Work out the finished part from the listing and answer in its coordinate system (mm). A direction names the side the tool comes from. Round coordinates to 2 decimals unless told otherwise and drop trailing zeros. Loops run counter-clockwise (first coordinate to the right, second up) from the corner with the lowest first, then second, coordinate; pieces in that order, holes last. Notation, with made-up numbers: (-6, -4.5) - (28, -4.5) arc R29 cw to (28, 17.5) - close; hole circle Ø11 at (55.25, 7). An arc over 180 degrees is marked (long way). Answer as CSV lines item,"result". Start each with the question number.
Q1. Each of these flat-tipped pins is pushed along its axis until it touches: pin 1 Ø4 at (x, y) = (35.15, 35.15) entering from +Z; pin 2 Ø1.7 at (x, y) = (14.63, -8.44) entering from -Z. Where does it stop, or does it pass through?
Q2. Section A-A on y = 9 is taken. Write down the section's boundary in (x, z), then the cut area to 3 significant figures.
Q3. Section B-B on x = -10 is taken. Write down the section's boundary in (y, z), then the cut area to 3 significant figures.
Q4. For faces 1 (the face through (-24.041, -17.546, 0.805)), 2 (the face through (-1, 1, 0)), determine the directions among +Z, -Z, +X, -X, +Y, -Y from which every point of the face is accessible in a straight line to the end or side of a thin tool.
Q5. Straight lines are drawn through the part: L1, parallel to Y at x = 0, z = 1; L2, parallel to Y at x = 7, z = 0.1; L3, parallel to X at y = 8.5, z = 1.4. For each, find the intervals that lie inside material, in ascending order. Write a range as [from, to].
Q6. Section D-D on y = -50 is taken. Write down the section's boundary in (x, z).
Q7. Section C-C on z = 1.1 is taken. Count the separate pieces of the cut face and the enclosed holes in it, then the cut area to 3 significant figures.
Q8. The mould has two halves that part along Y. Classify faces 3 (the face through (32.567, -57.397, 0.783)), 4 (the face through (-1, 1, 1.588)), 5 (the face through (0.18, -17.78, 0.8)): +Y half, -Y half, draft (parallel to the pull), parting line (faces both ways), or undercut.
```python
from build123d import *

# Parameters (mm, degrees)
F0_R            = 1.2192
F1_DEPTH        = 1.5875
F2_R            = 1.0922
F3_DEPTH        = 1.5875
F3_COPIES_COUNT = 3
F4_R            = 4.7625


# Not quite as in the source:
# - a pattern or mirror of a feature is missing from the dataset's text; its kind, count and spacing are read off the source's solid


with BuildPart() as f1:
    # F0 (on Top) → F1 (new body)
    with BuildSketch(Plane.XY):
        Polygon((65.9911357684, -38.1), (65.9911357684, 38.1), (0, 76.2), (-65.9911357684, 38.1), (-65.9911357684, -38.1), (0, -76.2), align=None)
        with Locations((-35.1536, -35.1536)):
            Circle(F0_R, mode=Mode.SUBTRACT)
        with Locations((35.1536, -35.1536)):
            Circle(F0_R, mode=Mode.SUBTRACT)
        with Locations((-35.1536, 35.1536)):
            Circle(F0_R, mode=Mode.SUBTRACT)
        with Locations((35.1536, 35.1536)):
            Circle(F0_R, mode=Mode.SUBTRACT)
    extrude(amount=F1_DEPTH)

    # F2 (on face) → F3 (cut, through all)
    with BuildSketch(Plane.XY.offset(1.5875)):
        with BuildLine():
            ThreePointArc((11.8486437632, -13.2566225326), (0, -17.78), (-11.8486437632, -13.2566225326))
            ThreePointArc((-11.8486437632, -13.2566225326), (-14.3916795622, -13.9960432527), (-16.9881251543, -13.4742728402))
            Line((-16.9881251543, -13.4742728402), (-31.2933003438, -21.7333695867))
            ThreePointArc((-31.2933003438, -21.7333695867), (0, -38.1), (31.2933003438, -21.7333695867))
            Line((31.2933003438, -21.7333695867), (16.9881251543, -13.4742728402))
            ThreePointArc((16.9881251543, -13.4742728402), (14.3916795622, -13.9960432527), (11.8486437632, -13.2566225326))
        make_face()
        with Locations((14.6267687632, -8.4447688828)):
            Circle(F2_R)
        with Locations((-14.6267687632, -8.4447688828)):
            Circle(F2_R)
    f3 = extrude(amount=-F3_DEPTH, mode=Mode.SUBTRACT)

    # F3_copies: F3 ×3 about axis
    f3_copies_axis = Axis((0, 0, 0), (0, 0, 1))
    for i in range(1, F3_COPIES_COUNT):
        add(f3.rotate(f3_copies_axis, i * 360 / F3_COPIES_COUNT), mode=Mode.SUBTRACT)

    # F4
    f4_edges = [f1.edges().sort_by_distance(p)[0] for p in [
        (-65.991136, 38.1, 0.79375),
        (0, 76.2, 0.79375),
        (65.991136, 38.1, 0.79375),
        (65.991136, -38.1, 0.79375),
        (0, -76.2, 0.79375),
        (-65.991136, -38.1, 0.79375),
    ]]
    fillet(f4_edges, radius=F4_R)


solid = f1.part
```
Findings:
1,pin 1,"stops at z = 1.59"
1,pin 2,"passes through"
2,outline,"(-65.99, 0) - (-37.02, 0) - (-37.02, 1.59) - (-65.99, 1.59) - close; (-15.33, 0) - (15.33, 0) - (15.33, 1.59) - (-15.33, 1.59) - close; (37.02, 0) - (65.99, 0) - (65.99, 1.59) - (37.02, 1.59) - close"
2,area,"141 mm^2"
3,outline,"(-70.43, 0) - (-36.76, 0) - (-36.76, 1.59) - (-70.43, 1.59) - close; (-14.7, 0) - (14.7, 0) - (14.7, 1.59) - (-14.7, 1.59) - close; (36.76, 0) - (70.43, 0) - (70.43, 1.59) - (36.76, 1.59) - close"
3,area,"154 mm^2"
4,face 1,"+Z, -Z"
4,face 2,"-Z, +X, -X, +Y, -Y"
5,L1,"y = [-75.46, -38.1], [-17.78, 15.8], [17.98, 75.46]"
5,L2,"y = [-72.16, -37.45], [-16.34, 16.34], [37.45, 72.16]"
5,L3,"x = [-65.99, -37.14], [-15.62, 15.62], [37.14, 65.99]"
6,outline,"(-45.38, 0) - (45.38, 0) - (45.38, 1.59) - (-45.38, 1.59) - close"
7,separate pieces,"1"
7,enclosed holes,"10"
7,area,"11,900 mm^2"
8,face 3,"-Y half"
8,face 4,"draft"
8,face 5,"undercut"
